```python
from build123d import *

# Parameters (mm, degrees)
EXTRUDE_1_DEPTH     = 22.5
SKETCH_2_R          = 1
CUT_EXTRUDE_1_DEPTH = 4


with BuildPart() as part:
    # 草图1 → 凸台-拉伸1 (new body)
    with BuildSketch(Plane(origin=(0, 0, 0), x_dir=(1, 0, 0), z_dir=(0, 1, 0))):
        Polygon((-3.5, -0.75), (3.5, -0.75), (3.5, 3.25), (8.5, 3.25), (8.5, -3.25), (-8.5, -3.25), (-8.5, 3.25), (-3.5, 3.25), align=None)
    extrude(amount=EXTRUDE_1_DEPTH)

    # 草图2 → 切除-拉伸1 (cut)
    with BuildSketch(Plane.XY.offset(3.25)):
        with Locations((-6, 15.5)):
            Circle(SKETCH_2_R)
        with Locations((-6, 7.5)):
            Circle(SKETCH_2_R)
        with Locations(Location((6, 7.5, 0), (0, 0, 180))):
            Circle(SKETCH_2_R)
        with Locations(Location((6, 15.5, 0), (0, 0, 180))):
            Circle(SKETCH_2_R)
    extrude(amount=-CUT_EXTRUDE_1_DEPTH, mode=Mode.SUBTRACT)


solid = part.part
```
Build history of the part. All positions in model axes, mm. A direction names the side the tool comes from. Round coordinates to 2 decimals unless told otherwise and drop trailing zeros. Write each loop counter-clockwise with the first axis right and the second up, starting at its lowest first coordinate (ties: lowest second). Pieces come first, ordered by that corner, then holes.
1) Band-saw the part on A-A, the plane z = -1. List the corners of the cut face in (x, y).
2) Pin check, flat tips, straight feed: pin 1 (0.6 mm diameter, centred on x = 5.5, y = 15.5, fed in from +Z); pin 2 (2 mm diameter, centred on x = -0.5, y = 15.5, fed in from -Z). Stop position of each tip, or through.
3) Band-saw the part on D-D, the plane z = 2. List the corners of the cut face in (x, y), and give its area (3 significant figures).
4) Band-saw the part on B-B, the plane x = -6. List the corners of the cut face in (y, z).
5) Drill centre lines: probe 1 along Y at (x, z) = (-6, 1.45); probe 2 along X at (y, z) = (15, 2.5); probe 3 along X at (y, z) = (12.25, 0.25). Where is each one in solid material? Low to high.
6) 3-axis set-ups, long thin cutter, end or side, ignore diameter. For faces 4 (the flat face through (-3.5, 11, -1)), 5 (the cylindrical face through (-6.13, 8.49, 1.28)), 6 (the flat face through (8.5, 11, 0)): which of +Z, -Z, +X, -X, +Y, -Y reach the whole face in a straight line?
7) Mould opens along X. For faces 1 (the flat face through (6, 11, -3.25)), 2 (the cylindrical face through (-6.217, 14.524, 1.278)), 3 (the flat face through (-8.5, 11, 0)) say: +X half, -X half, draft (parallel to the pull), parting line (faces both ways), or undercut.
8) Band-saw the part on C-C, the plane y = 15.5. List the corners of the cut face in (x, z), and give its area (3 significant figures).
Ans:
1. outline: (-8.5, 0) - (-3.5, 0) - (-3.5, 22.5) - (-8.5, 22.5) - close; (3.5, 0) - (8.5, 0) - (8.5, 22.5) - (3.5, 22.5) - close
2. pin 1: stops at z = -0.75
2. pin 2: stops at z = 0.75
3. outline: (-8.5, 0) - (8.5, 0) - (8.5, 22.5) - (-8.5, 22.5) - close; hole circle Ø2 at (-6, 7.5); hole circle Ø2 at (-6, 15.5); hole circle Ø2 at (6, 7.5); hole circle Ø2 at (6, 15.5)
3. area: 370 mm2
4. outline: (0, -3.25) - (22.5, -3.25) - (22.5, 3.25) - (16.5, 3.25) - (16.5, -0.75) - (14.5, -0.75) - (14.5, 3.25) - (8.5, 3.25) - (8.5, -0.75) - (6.5, -0.75) - (6.5, 3.25) - (0, 3.25) - close
5. probe 1: y = 0 to 6.5, 8.5 to 14.5, 16.5 to 22.5
5. probe 2: x = -8.5 to -6.87, -5.13 to 5.13, 6.87 to 8.5
5. probe 3: x = -8.5 to -3.5, 3.5 to 8.5
6. face 4: -Z, +Y, -Y
6. face 5: +Z
6. face 6: +Z, -Z, +X, +Y, -Y
7. face 1: draft
7. face 2: undercut
7. face 3: -X half
8. outline: (-8.5, -3.25) - (-3.5, -3.25) - (-3.5, 0.75) - (3.5, 0.75) - (3.5, -3.25) - (8.5, -3.25) - (8.5, 3.25) - (7, 3.25) - (7, -0.75) - (5, -0.75) - (5, 3.25) - (-5, 3.25) - (-5, -0.75) - (-7, -0.75) - (-7, 3.25) - (-8.5, 3.25) - close
8. area: 66.5 mm2
